Source: CAD feature listing. Evaluate the final solid. Frame: model axes, mm. A direction names the side the tool comes from. Round coordinates to 2 decimals unless told otherwise and drop trailing zeros. Loops run counter-clockwise (first coordinate to the right, second up) from the corner with the lowest first, then second, coordinate; pieces in that order, holes last.
(1) Material intervals for probe 1 along Y at (x, z) = (0, 2.25); probe 2 along Z at (x, y) = (-4.25, -3.5); probe 3 along Y at (x, z) = (-2.5, 1.45), sorted ascending.
(2) Section C-C, the plane z = 2.35. Return the cut outline in (x, y).
(3) Set-up query: faces 4 (the cylindrical face through (4.91, 1.55, 1.97)), 5 (the cylindrical face through (-1.28, -5.76, 4.48)). Return all of +Z, -Z, +X, -X, +Y, -Y with unobstructed straight access to the full face (end or side cutting, diameter ignored); none if empty.
(4) Section A-A, the plane x = 0. Return the cut outline in (y, z).
(5) First-contact query: pin 1 Ø1.5 at (x, z) = (-4, 1) entering from -Y; pin 2 Ø1 at (x, z) = (1.5, 1) entering from -Y. Flat tips, straight axial feed; report the tip coordinate or a pass-through.
(6) Mould query, pull axis Y, two halves, no side actions, for faces 1 (the cylindrical face through (-1.38, -6.2, 2.22)), 2 (the flat face through (-2, 5, 4)), 3 (the flat face through (-2, 5, 0)). Classes: pulls with the +Y half, pulls with the -Y half, needs draft (parallel to the pull), parting line crosses it, or undercut.
```python
from build123d import *

# Parameters (mm, degrees)
F0_R     = 6.35
F0_R_2   = 5.15
F1_DEPTH = 5
F2_R     = 5.9
F2_R_2   = 5.15
F3_DEPTH = 1


# Not quite as in the source:
# - a fillet or chamfer that OpenCascade refuses, or shapes differently, is made with other operations: its cross-section is extruded or revolved along the edge and cut away or added


with BuildPart() as f1:
    # F0 (on Top) → F1 (new body)
    with BuildSketch(Plane.XY):
        Circle(F0_R)
        Circle(F0_R_2, mode=Mode.SUBTRACT)
    extrude(amount=F1_DEPTH)

    # F2 (on face) → F3 (cut)
    with BuildSketch(Plane.XY.offset(5)):
        Circle(F2_R)
        Circle(F2_R_2, mode=Mode.SUBTRACT)
    extrude(amount=-F3_DEPTH, mode=Mode.SUBTRACT)

    # F4: chamfer of 0.5 on 1 edges, made by hand

    # F4_s1 → F4_t2 (revolve, cut)
    with BuildSketch(Plane.XZ):
        Polygon((6.35, 4.5), (5.85, 5), (6.35, 5), align=None)
    revolve(axis=Axis((0, 0, 5), (0, 0, 1)), mode=Mode.SUBTRACT)


solid = f1.part
```
Output values:
1. probe 1: y = -6.35 to -5.15, 5.15 to 6.35
1. probe 2: z = 0 to 4
1. probe 3: y = -5.84 to -4.5, 4.5 to 5.84
2. outline: circle Ø12.7 at (0, 0); hole circle Ø10.3 at (0, 0)
3. face 4: +Z, -Z
3. face 5: +Z
4. outline: (-6.35, 0) - (-5.15, 0) - (-5.15, 4) - (-5.9, 4) - (-5.9, 4.95) - (-6.35, 4.5) - close; (5.15, 0) - (6.35, 0) - (6.35, 4.5) - (5.9, 4.95) - (5.9, 4) - (5.15, 4) - close
5. pin 1: stops at y = -5.46
5. pin 2: stops at y = -6.27
6. face 1: parting line crosses it
6. face 2: undercut
6. face 3: needs draft
